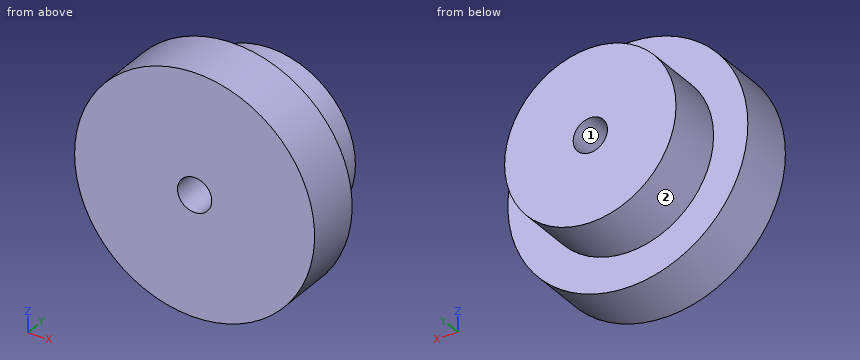
Autodesk Inventor part; units mm, degrees
ref_plane "YZ Plane" through (0, 0, 0) normal (1, 0, 0) x (0, 1, 0)
ref_plane "XZ Plane" through (0, 0, 0) normal (0, 1, 0) x (-1, 0, 0)
ref_plane "XY Plane" through (0, 0, 0) normal (0, 0, 1) x (1, 0, 0)
sketch "Sketch1" plane through (0, 0, 0) normal (0, 1, 0) x (-1, 0, 0)
  circle A0 centre (0, 0) radius 10.5
  dimension "d0" = 21
extrude "Extrusion1" add sketch "Sketch1" along normal blind 5
sketch "Sketch2" plane through (0, 5, 0) normal (0, 1, 0) x (1, 0, 0)
  circle A0 centre (0, 0) radius 7.5
  dimension "d3" = 15
extrude "Extrusion2" add sketch "Sketch2" along normal blind 5
sketch "Sketch3" plane through (0, 10, 0) normal (0, 1, 0) x (1, 0, 0)
  circle A0 centre (0, 0) radius 1.5
  dimension "d6" = 3
extrude "Extrusion3" cut sketch "Sketch3" against normal through all
properties part number "Gear" material "Brass, Soft Yellow"
Geometry: final body of the model. Coordinates: model frame, mm. Face numbers are marked on the shaded views. A direction names the side the tool comes from. Coordinates: 2 decimals unless noted, no trailing zeros. Order: outer loops, then holes, each group sorted by start corner. A loop starts at its lowest first (then second) coordinate and runs counter-clockwise, first axis right, second up.
(1) Section query B-B (z = 0). Return the cut outline in (x, y).
(2) Material intervals for probe 1 along Z at (x, y) = (0, 7); probe 2 along Z at (x, y) = (0, 4), sorted ascending.
(3) Section query C-C (y = 1.25). Return the cut outline in (x, z), plus the area to 3 significant figures.
(4) First-contact query: pin 1 (1 mm diameter, centred on x = 1, y = 7, fed in from -Z); pin 2 (2 mm diameter, centred on y = 3.5, z = 5.5, fed in from +X); pin 3 (5 mm diameter, centred on x = 0, z = 0, fed in from -Y); pin 4 (6 mm diameter, centred on x = -7.5, y = 4.5, fed in from -Z). Flat tips, straight axial feed; report the tip coordinate or a pass-through.
(5) Access query for the marked faces 1 and 2. Directions: +Z, -Z, +X, -X, +Y, -Y. A direction counts if a zero-diameter tool reaches every point of the face in a straight line with its end or side. Return the directions, or none.
(6) Section query D-D (x = 5). Return the cut outline in (y, z), plus the area to 3 significant figures.
(7) Section query A-A (x = 0). Return the cut outline in (y, z).
Solution:
1. outline: (-10.5, 0) - (-1.5, 0) - (-1.5, 10) - (-7.5, 10) - (-7.5, 5) - (-10.5, 5) - close; (1.5, 0) - (10.5, 0) - (10.5, 5) - (7.5, 5) - (7.5, 10) - (1.5, 10) - close
2. probe 1: z = -7.5 to -1.5, 1.5 to 7.5
2. probe 2: z = -10.5 to -1.5, 1.5 to 10.5
3. outline: circle Ø21 at (0, 0); hole circle Ø3 at (0, 0)
3. area: 339 mm2
4. pin 1: stops at z = -7.48
4. pin 2: stops at x = 9.49
4. pin 3: stops at y = 0
4. pin 4: stops at z = -9.49
5. face 1: +Y, -Y
5. face 2: +Y
6. outline: (0, -9.23) - (5, -9.23) - (5, -5.59) - (10, -5.59) - (10, 5.59) - (5, 5.59) - (5, 9.23) - (0, 9.23) - close
6. area: 148 mm2
7. outline: (0, -10.5) - (5, -10.5) - (5, -7.5) - (10, -7.5) - (10, -1.5) - (0, -1.5) - close; (0, 1.5) - (10, 1.5) - (10, 7.5) - (5, 7.5) - (5, 10.5) - (0, 10.5) - close
